```python
from build123d import *

# Parameters (mm, degrees)
SKETCH1_W           = 120
SKETCH1_H           = 65
SKETCH1_R           = 1.7
SKETCH1_R_2         = 3.05
SKETCH1_R_3         = 2.5
BOSS_EXTRUDE1_DEPTH = 10
SKETCH2_R           = 5
CUT_EXTRUDE1_DEPTH  = 6


with BuildPart() as part:
    # Sketch1 → Boss-Extrude1 (new body)
    with BuildSketch(Plane.XY):
        with Locations((60, 32.5)):
            Rectangle(SKETCH1_W, SKETCH1_H)
        with Locations((85, 7.5)):
            Circle(SKETCH1_R, mode=Mode.SUBTRACT)
        with Locations((85, 57.5)):
            Circle(SKETCH1_R, mode=Mode.SUBTRACT)
        with Locations((35, 7.5)):
            Circle(SKETCH1_R, mode=Mode.SUBTRACT)
        with Locations((35, 57.5)):
            Circle(SKETCH1_R, mode=Mode.SUBTRACT)
        with Locations((110, 7.5)):
            Circle(SKETCH1_R_2, mode=Mode.SUBTRACT)
        with Locations((110, 57.5)):
            Circle(SKETCH1_R_2, mode=Mode.SUBTRACT)
        with Locations((10, 7.5)):
            Circle(SKETCH1_R_2, mode=Mode.SUBTRACT)
        with Locations((10, 57.5)):
            Circle(SKETCH1_R_2, mode=Mode.SUBTRACT)
        with Locations((110, 32.5)):
            Circle(SKETCH1_R_3, mode=Mode.SUBTRACT)
        with Locations((10, 32.5)):
            Circle(SKETCH1_R_3, mode=Mode.SUBTRACT)
    extrude(amount=BOSS_EXTRUDE1_DEPTH)

    # Sketch2 → Cut-Extrude1 (cut)
    with BuildSketch(Plane.XY.offset(10)):
        with Locations((110, 7.5)):
            Circle(SKETCH2_R)
        with Locations((110, 57.5)):
            Circle(SKETCH2_R)
        with Locations((10, 57.5)):
            Circle(SKETCH2_R)
        with Locations((10, 7.5)):
            Circle(SKETCH2_R)
    extrude(amount=-CUT_EXTRUDE1_DEPTH, mode=Mode.SUBTRACT)


solid = part.part
```
Read the model definition and answer for the solid it produces. Units are mm, in the model's axes. A direction names the side the tool comes from. Give positions to 0.01 mm unless a question says otherwise; leave off trailing zeros. Order: outer loops, then holes, each group sorted by start corner. A loop starts at its lowest first (then second) coordinate and runs counter-clockwise, first axis right, second up. Notation, with made-up numbers: (-19, 83.5) -> (19, 83.5) arc R23 ccw to (19, 120.5) -> close; hole circle Ø7 at (9, 25). An arc over 180 degrees is marked (long way). One line per item, written item: value. Start each with the question number.
(1) Flat-ended cylindrical pins translate along their axes: P1, Ø5, axis at x = 109.5, y = 56, coming from the +Z side; P2, Ø5.5, axis at x = 10, y = 7.5, coming from the -Z side. Find the tip coordinate at first contact, or state that the pin passes through.
(2) The part is cut by section D-D (z = 5.5). State how many separate pieces and enclosed holes the cut face has, and give its area (3 significant figures).
(3) The part is cut by section A-A (x = 85). Determine the outline of the cut face in (y, z), and give its area (3 significant figures).
(4) The part is cut by section B-B (x = 10). Determine the outline of the cut face in (y, z), and give its area (3 significant figures).
(5) Straight lines are drawn through the part: L1, parallel to Y at x = 110, z = 2; L2, parallel to Y at x = 110, z = 7.9; L3, parallel to X at y = 55, z = 3.5. For each, find the intervals that lie inside material, in ascending order.
(6) For a pull along Y with two mould halves and no side action, classify faces 3 (the flat face through (59, 33, 0)), 4 (the flat face through (59, 0, 5)), 5 (the cylindrical face through (11.34, 34.61, 4.93)), 6 (the cylindrical face through (106.953, 7.634, 1.972)) as released by +Y, released by -Y, zero draft, split by the parting line, or undercut.
(7) A tool of negligible diameter and unlimited length cuts with its end or side. For faces 1 (the flat face through (112, 10, 4)), 2 (the flat face through (59, 33, 10)), from which of +Z, -Z, +X, -X, +Y, -Y can it reach the whole face along a straight path? Write none if from no direction.
(8) The part is cut by section C-C (y = 7.5). Determine the outline of the cut face in (x, z).
Taken from the geometry:
1. P1: z = 4
1. P2: through
2. separate pieces: 1
2. enclosed holes: 10
2. area: 7,410 mm^2
3. outline: (0, 0) -> (5.8, 0) -> (5.8, 10) -> (0, 10) -> close; (9.2, 0) -> (55.8, 0) -> (55.8, 10) -> (9.2, 10) -> close; (59.2, 0) -> (65, 0) -> (65, 10) -> (59.2, 10) -> close
3. area: 582 mm^2
4. outline: (0, 0) -> (4.45, 0) -> (4.45, 4) -> (2.5, 4) -> (2.5, 10) -> (0, 10) -> close; (10.55, 0) -> (30, 0) -> (30, 10) -> (12.5, 10) -> (12.5, 4) -> (10.55, 4) -> close; (35, 0) -> (54.45, 0) -> (54.45, 4) -> (52.5, 4) -> (52.5, 10) -> (35, 10) -> close; (60.55, 0) -> (65, 0) -> (65, 10) -> (62.5, 10) -> (62.5, 4) -> (60.55, 4) -> close
4. area: 431 mm^2
5. L1: 0 to 4.45, 10.55 to 30, 35 to 54.45, 60.55 to 65
5. L2: 0 to 2.5, 12.5 to 30, 35 to 52.5, 62.5 to 65
5. L3: 0 to 8.25, 11.75 to 108.25, 111.75 to 120
6. face 3: zero draft
6. face 4: released by -Y
6. face 5: undercut
6. face 6: undercut
7. face 1: +Z
7. face 2: +Z, +X, -X, +Y, -Y
8. outline: (0, 0) -> (6.95, 0) -> (6.95, 4) -> (5, 4) -> (5, 10) -> (0, 10) -> close; (13.05, 0) -> (33.3, 0) -> (33.3, 10) -> (15, 10) -> (15, 4) -> (13.05, 4) -> close; (36.7, 0) -> (83.3, 0) -> (83.3, 10) -> (36.7, 10) -> close; (86.7, 0) -> (106.95, 0) -> (106.95, 4) -> (105, 4) -> (105, 10) -> (86.7, 10) -> close; (113.05, 0) -> (120, 0) -> (120, 10) -> (115, 10) -> (115, 4) -> (113.05, 4) -> close
